```python
from build123d import *

# Parameters (mm, degrees)
CROQUIS1_W              = 55
CROQUIS1_H              = 15
CROQUIS1_R              = 1.175
CROQUIS1_R_2            = 1.185
CROQUIS1_R_3            = 1.195
CROQUIS1_R_4            = 1.205
CROQUIS1_R_5            = 1.215
CROQUIS1_R_6            = 1.225
CROQUIS1_R_7            = 1.235
CROQUIS1_R_8            = 1.245
CROQUIS1_R_9            = 1.255
CROQUIS1_R_10           = 1.265
CROQUIS1_R_11           = 1.275
SALIENTE_EXTRUIR1_DEPTH = 3


with BuildPart() as part:
    # Croquis1 → Saliente-Extruir1 (new body)
    with BuildSketch(Plane(origin=(0, 0, 0), x_dir=(1, 0, 0), z_dir=(0, 1, 0))):
        Rectangle(CROQUIS1_W, CROQUIS1_H)
        with Locations(Location((-21.88537105, 0, 0), (0, 0, 270))):
            Circle(CROQUIS1_R, mode=Mode.SUBTRACT)
        with Locations(Location((-17.678607244, 0, 0), (0, 0, 270))):
            Circle(CROQUIS1_R_2, mode=Mode.SUBTRACT)
        with Locations(Location((-13.4135496, 0, 0), (0, 0, 270))):
            Circle(CROQUIS1_R_3, mode=Mode.SUBTRACT)
        with Locations(Location((-9.099468305, 0, 0), (0, 0, 270))):
            Circle(CROQUIS1_R_4, mode=Mode.SUBTRACT)
        with Locations(Location((-4.295150499, 0, 0), (0, 0, 270))):
            Circle(CROQUIS1_R_5, mode=Mode.SUBTRACT)
        with Locations(Location((0, 0, 0), (0, 0, 270))):
            Circle(CROQUIS1_R_6, mode=Mode.SUBTRACT)
        with Locations(Location((4.921295904, 0, 0), (0, 0, 270))):
            Circle(CROQUIS1_R_7, mode=Mode.SUBTRACT)
        with Locations(Location((9.643654095, 0, 0), (0, 0, 270))):
            Circle(CROQUIS1_R_8, mode=Mode.SUBTRACT)
        with Locations(Location((14.38652568, 0, 0), (0, 0, 270))):
            Circle(CROQUIS1_R_9, mode=Mode.SUBTRACT)
        with Locations(Location((19.028560127, 0, 0), (0, 0, 270))):
            Circle(CROQUIS1_R_10, mode=Mode.SUBTRACT)
        with Locations(Location((23.245310452, 0, 0), (0, 0, 270))):
            Circle(CROQUIS1_R_11, mode=Mode.SUBTRACT)
    extrude(amount=SALIENTE_EXTRUIR1_DEPTH)


solid = part.part
```
Can you work these out from the model? Positions are in its coordinate system, mm. Give positions to 0.01 mm unless a question says otherwise; leave off trailing zeros. Order: outer loops, then holes, each group sorted by start corner. A loop starts at its lowest first (then second) coordinate and runs counter-clockwise, first axis right, second up. Notation, with made-up numbers: M -20.5,-8 L 27.5,-8 A19 cw 27.5,15 Z; hole C 84,11.5 d3. An arc over 180 degrees is marked long. Write item = value, one per line. Start each with the question number.
Q1. Suppose I cut it at A-A (x = 0). Write out the boundary of the cut face in (y, z) (3 decimals).
Q2. I need wall thicknesses on probe 1 along Z at (x, y) = (-5, 2); probe 2 along Z at (x, y) = (-10, 1.8). Which ranges of each line are inside material? Lowest first, please. Write a range as [from, to].
Q3. We'd pull the mould along Z, two halves only. Please class faces 1 (the flat face through (0, 3, -2)), 2 (the flat face through (0, 1, -7.5)), 3 (the cylindrical face through (8.9, 1.5, -1)): pulls with the +Z half, pulls with the -Z half, needs draft (parallel to the pull), parting line crosses it, or undercut.
Q4. Suppose I cut it at B-B (z = 0). Count the separate pieces of the cut face and the enclosed holes in it, plus the area to 4 significant figures.
Q5. Will this pin go through, and if not, where does the flat tip stop? pin 1 Ø1.5 at (x, z) = (0, 0) entering from -Y.
Check result:
q1.outline = M 0,-7.5 L 3,-7.5 L 3,-1.225 L 0,-1.225 Z; M 0,1.225 L 3,1.225 L 3,7.5 L 0,7.5 Z
q2.probe_1 = [-7.5, -0.99], [0.99, 7.5]
q2.probe_2 = [-7.5, -0.8], [0.8, 7.5]
q3.face_1 = needs draft
q3.face_2 = pulls with the -Z half
q3.face_3 = undercut
q4.separate_pieces = 12
q4.enclosed_holes = 0
q4.area = 84.15 mm2
q5.pin_1 = through
